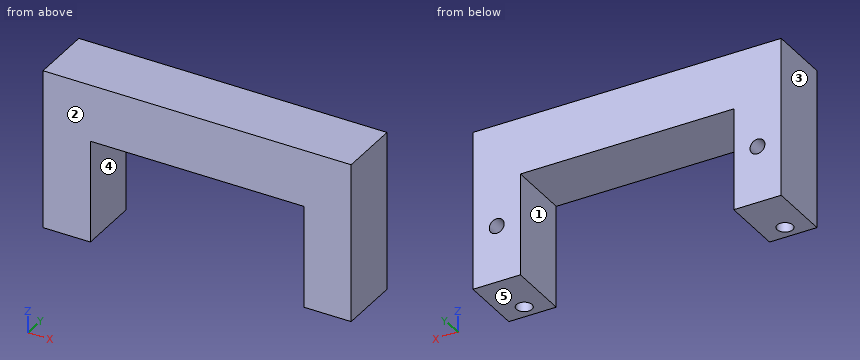
from build123d import *

# Parameters (mm, degrees)
F1_DEPTH      = 10.668
F2_W          = 2.54
F2_H          = 13.716
F2_W_2        = 10.541
F3_DEPTH      = 20.6385
F3_DEPTH_BACK = 20.6385
F4_R          = 1
F5_DEPTH      = 5.08
F6_R          = 1.05
F7_DEPTH      = 6.985
F8_W          = 11.4453516792
F8_H          = 8.6245518178
F8_W_2        = 4.2650750415
F9_DEPTH      = 20.6385
F9_DEPTH_BACK = 20.6385


with BuildPart() as f1:
    # F0 (on Front) → F1 (new body, symmetric)
    with BuildSketch(Plane.XZ):
        Polygon((-14.2875, 0), (0, 0), (14.2875, 0), (14.2875, -13.716), (20.6375, -13.716), (20.6375, 7.62), (0, 7.62), (-20.6375, 7.62), (-20.6375, -13.716), (-14.2875, -13.716), align=None)
    extrude(amount=F1_DEPTH, both=True)

    # F2 (on Right) → F3 (cut, two sides)
    with BuildSketch(Plane.YZ) as f3_sk:
        with Locations((9.398, -6.858)):
            Rectangle(F2_W, F2_H)
        with Locations((-5.3975, -6.858)):
            Rectangle(F2_W_2, F2_H)
    extrude(amount=-F3_DEPTH, mode=Mode.SUBTRACT)
    extrude(f3_sk.sketch, amount=F3_DEPTH_BACK, mode=Mode.SUBTRACT)

    # F4 (on face) → F5 (cut)
    with BuildSketch(Plane(origin=(0, 8.128, 0), x_dir=(-1, 0, 0), z_dir=(0, 1, 0))):
        with Locations((-17.4625, -6.096)):
            Circle(F4_R)
        with Locations((17.4625, -6.096)):
            Circle(F4_R)
    extrude(amount=-F5_DEPTH, mode=Mode.SUBTRACT)

    # F6 (on face) → F7 (cut)
    with BuildSketch(Plane(origin=(0, 0, -13.716), x_dir=(1, 0, 0), z_dir=(0, 0, -1))):
        with Locations((-17.4625, -1.778)):
            Circle(F6_R)
        with Locations((17.4625, -1.778)):
            Circle(F6_R)
    extrude(amount=-F7_DEPTH, mode=Mode.SUBTRACT)

    # F8 (on Right) → F9 (cut, two sides)
    with BuildSketch(Plane.YZ) as f9_sk:
        with Locations((-5.8496758396, 4.3122759089)):
            Rectangle(F8_W, F8_H)
        with Locations((10.2605375207, 4.3122759089)):
            Rectangle(F8_W_2, F8_H)
    extrude(amount=F9_DEPTH, mode=Mode.SUBTRACT)
    extrude(f9_sk.sketch, amount=-F9_DEPTH_BACK, mode=Mode.SUBTRACT)


solid = f1.part
Part model, mm, in its own coordinate system. Face numbers are marked on the shaded views. A direction names the side the tool comes from. Coordinates: 2 decimals unless noted, no trailing zeros. Write each loop counter-clockwise with the first axis right and the second up, starting at its lowest first coordinate (ties: lowest second). Pieces come first, ordered by that corner, then holes. Notation, with made-up numbers: M 3,72 L 58,72 A26 ccw 58,109 Z; hole C 70,28 d1. An arc over 180 degrees is marked long. Return JSON: item names as keys, results as strings.
1. 3-axis set-ups, long thin cutter, end or side, ignore diameter. For the marked faces 1 and 2: which of +Z, -Z, +X, -X, +Y, -Y reach the whole face in a straight line?
Determined:
{"face 1": "-Z, +Y, -Y", "face 2": "+Z, -Z, +X, -X, -Y"}
2. Pull direction X, two halves, no side cores. Call the marked faces 3, 4 and 5: pulls with the +X half, pulls with the -X half, needs draft (parallel to the pull), parting line crosses it, or undercut.
Determined:
{"face 3": "pulls with the -X half", "face 4": "undercut", "face 5": "needs draft"}
3. Flat gauge pins, fed straight in: pin 1 Ø1.9 at (x, y) = (17.46, 1.78) entering from -Z; pin 2 Ø2.5 at (x, z) = (17.46, -6.1) entering from +Y; pin 3 Ø1.2 at (x, z) = (-17.46, -6.1) entering from +Y; pin 4 Ø3 at (x, y) = (-3.5, 2) entering from -Z. Where does each tip first touch, or does it go through?
Determined:
{"pin 1": "z = -6.73", "pin 2": "y = 8.13", "pin 3": "y = 3.05", "pin 4": "z = 0"}
4. Saw through at A-A, the plane z = -4. Write the cut outline in (x, y).
Determined:
{"outline": "M -20.64,-0.13 L -14.29,-0.13 L -14.29,8.13 L -20.64,8.13 Z; M 14.29,-0.13 L 20.64,-0.13 L 20.64,8.13 L 14.29,8.13 Z"}
5. Saw through at C-C, the plane z = -7.75. Write the cut outline in (x, y).
Determined:
{"outline": "M -20.64,-0.13 L -14.29,-0.13 L -14.29,8.13 L -20.64,8.13 Z; M 14.29,-0.13 L 20.64,-0.13 L 20.64,8.13 L 14.29,8.13 Z; hole C -17.46,1.78 d2.1; hole C 17.46,1.78 d2.1"}
6. Saw through at D-D, the plane x = 18. Write the cut outline in (y, z).
Determined:
{"outline": "M -0.13,-13.72 L 0.88,-13.72 L 0.88,-6.73 L 2.68,-6.73 L 2.68,-13.72 L 8.13,-13.72 L 8.13,-6.94 L 3.05,-6.94 L 3.05,-5.25 L 8.13,-5.25 L 8.13,7.62 L -0.13,7.62 Z"}
7. Saw through at B-B, the plane y = 6.5. Write the cut outline in (x, z), then the cut area to 3 significant figures.
Determined:
{"outline": "M -20.64,-13.72 L -14.29,-13.72 L -14.29,0 L 14.29,0 L 14.29,-13.72 L 20.64,-13.72 L 20.64,7.62 L -20.64,7.62 Z; hole C -17.46,-6.1 d2; hole C 17.46,-6.1 d2", "area": "482 mm²"}
8. Probe L1, parallel to X at y = 7.5, z = -3; L2, parallel to X at y = 2.25, z = -7.25; L3, parallel to Z at x = -17, y = 6.25. List the from-to ranges inside material, lowest first.
Determined:
{"L1": "-20.64 to -14.29, 14.29 to 20.64", "L2": "-20.64 to -18.4, -16.52 to -14.29, 14.29 to 16.52, 18.4 to 20.64", "L3": "-13.72 to -6.98, -5.21 to 7.62"}
